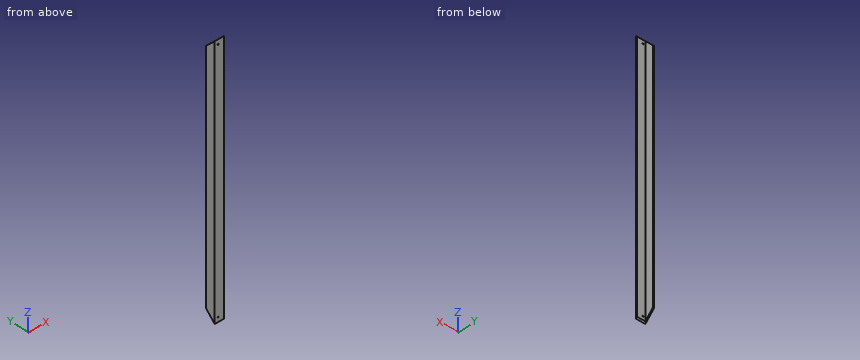
```python
from build123d import *

# Parameters (mm, degrees)
BOSS_EXTRUDE1_DEPTH = 704.85
CUT_EXTRUDE1_DEPTH  = 711.2
SKETCH3_R           = 1.5
CUT_EXTRUDE2_DEPTH  = 711.2


with BuildPart() as part:
    # Sketch1 → Boss-Extrude1 (new body)
    with BuildSketch(Plane.XY):
        Polygon((0, 25.4), (0, 0), (25.4, 0), (25.4, 3.175), (3.175, 3.175), (3.175, 25.4), align=None)
    extrude(amount=BOSS_EXTRUDE1_DEPTH)

    # Sketch2 → Cut-Extrude1 (cut)
    with BuildSketch(Plane.ZY):
        Polygon((0, 8.542079309), (0, 0), (25.4, 25.4), (0, 25.4), align=None)
        Polygon((704.85, 25.4), (679.45, 25.4), (704.85, 0), align=None)
    extrude(amount=-CUT_EXTRUDE1_DEPTH, mode=Mode.SUBTRACT)

    # Sketch3 → Cut-Extrude2 (cut)
    with BuildSketch(Plane.XZ):
        with Locations((9.525, 692.15)):
            Circle(SKETCH3_R)
        with Locations((9.525, 12.7)):
            Circle(SKETCH3_R)
    extrude(amount=-CUT_EXTRUDE2_DEPTH, mode=Mode.SUBTRACT)


solid = part.part
```
Verification items for the finished model (mm, model axes). Coordinates: 2 decimals unless noted, no trailing zeros. Write each loop counter-clockwise with the first axis right and the second up, starting at its lowest first coordinate (ties: lowest second). Pieces come first, ordered by that corner, then holes. Notation, with made-up numbers: M 31,38.5 L 46,38.5 A21 ccw 46,70.5 Z; hole C 41.5,27 d11. An arc over 180 degrees is marked long. One line per item, written item: value.
Item 1: Section check B-B, the plane y = 19.75. Record the boundary of the cut face in (x, z) (3 decimals).
Check sheet entries:
outline: M 0,19.75 L 3.175,19.75 L 3.175,685.1 L 0,685.1 Z
Item 2: Section check A-A, the plane z = 513.5. Record the boundary of the cut face in (x, y) (3 decimals).
Check sheet entries:
outline: M 0,0 L 25.4,0 L 25.4,3.175 L 3.175,3.175 L 3.175,25.4 L 0,25.4 Z
Item 3: Scan lines: line 1 along X through (y, z) = (0.7, 692.15) (3 decimals); line 2 along Y through (x, z) = (22.25, 231.5) (3 decimals). Record each from-to range of solid material in increasing order.
Check sheet entries:
line 1: x = 0 to 8.025, 11.025 to 25.4
line 2: y = 0 to 3.175
Item 4: Section check C-C, the plane x = 15. Record the boundary of the cut face in (y, z) (3 decimals), plus the area to 3 significant figures.
Check sheet entries:
outline: M 0,0 L 3.175,3.175 L 3.175,701.675 L 0,704.85 Z
area: 2,230 mm^2
Item 5: Gauge pin test, flat ends, axial feed: pin 1 Ø4 at (y, z) = (12.5, 599) entering from +X (3 decimals); pin 2 Ø2.5 at (x, z) = (9.525, 12.7) entering from +Y; pin 3 Ø4 at (x, z) = (9.525, 692.15) entering from +Y (3 decimals). Record the tip position at first contact, or that the pin passes through.
Check sheet entries:
pin 1: stops at x = 3.175
pin 2: passes through
pin 3: stops at y = 3.175
